The listing builds one solid part. Answer for the finished solid, in the listing's coordinates (mm). A direction names the side the tool comes from. Round coordinates to 2 decimals unless told otherwise and drop trailing zeros. Write each loop counter-clockwise with the first axis right and the second up, starting at its lowest first coordinate (ties: lowest second). Pieces come first, ordered by that corner, then holes. Notation, with made-up numbers: (-1.75, 72.25) - (21.25, 72.25) arc R6 cw to (21.25, 77.25) - close; hole circle Ø9 at (-17.5, 67). An arc over 180 degrees is marked (long way). Answer in a Markdown table with one row per item.
from build123d import *
from OCP.BRepFilletAPI import BRepFilletAPI_MakeChamfer

# Parameters (mm, degrees)
EXTRUDE_1_DEPTH         = 8
CHAMFER_12_SIZE         = 7
CHAMFER_12_SIZE2        = 5
HOLE_WIZARD_M2_22_D     = 2.3
HOLE_WIZARD_M2_22_DEPTH = 3.5
HOLE_WIZARD_M2_22_TIP   = 0.690989712
SKETCH_11_R             = 30
CUT_EXTRUDE_1_DEPTH     = 1.5
EXTRUDE_5_DEPTH         = 8
EXTRUDE_5_2_DEPTH       = 8
EXTRUDE_5_3_DEPTH       = 8
EXTRUDE_5_4_DEPTH       = 8
CHAMFER_13_SIZE         = 5
CHAMFER_13_SIZE2        = 7
CHAMFER_14_SIZE         = 5
CHAMFER_14_SIZE2        = 7
CHAMFER_15_SIZE         = 7
CHAMFER_15_SIZE2        = 5
CHAMFER_16_SIZE         = 5
CHAMFER_16_SIZE2        = 7
SKETCH_23_W             = 32
SKETCH_23_H             = 72
CUT_EXTRUDE_7_DEPTH     = 1.5
SKETCH_13_W             = 16
SKETCH_13_H             = 24
CUT_EXTRUDE_2_DEPTH     = 1.5


with BuildPart() as part:
    # Эскиз1 → Бобышка-Вытянуть1 (new body)
    with BuildSketch(Plane.XY):
        with BuildLine():
            Line((28.8, 21.6), (0, 60))
            Line((0, 60), (-28.8, 21.6))
            ThreePointArc((-28.8, 21.6), (-36, 0), (-28.8, -21.6))
            Line((-28.8, -21.6), (0, -60))
            Line((0, -60), (28.8, -21.6))
            ThreePointArc((28.8, -21.6), (36, 0), (28.8, 21.6))
        make_face()
        with BuildLine():
            ThreePointArc((4.1408267, 28.197580645), (0, -28.5), (-4.1408267, 28.197580645))
            ThreePointArc((-4.1408267, 28.197580645), (0, 26), (4.1408267, 28.197580645))
        make_face(mode=Mode.SUBTRACT)
    extrude(amount=EXTRUDE_1_DEPTH)

    # Фаска12: one chamfer whose edges measure the first distance from different faces: ONE call of the kernel's chamfer builder (chamfer() names one face for all edges)
    chamfer_12_edges_1 = [part.edges().sort_by_distance(p)[0] for p in [
        (14.4, 40.8, 0),
    ]]
    chamfer_12_side_1 = [part.faces().sort_by_distance(p)[0] for p in [
        (14.4, 40.8, 4),
    ]]
    chamfer_12_edges_2 = [part.edges().sort_by_distance(p)[0] for p in [
        (36, 0, 0),
    ]]
    chamfer_12_side_2 = [part.faces().sort_by_distance(p)[0] for p in [
        (36, 0, 4),
    ]]
    chamfer_12_edges_3 = [part.edges().sort_by_distance(p)[0] for p in [
        (14.4, -40.8, 0),
    ]]
    chamfer_12_side_3 = [part.faces().sort_by_distance(p)[0] for p in [
        (14.4, -40.8, 4),
    ]]
    chamfer_12_edges_4 = [part.edges().sort_by_distance(p)[0] for p in [
        (-14.4, -40.8, 0),
    ]]
    chamfer_12_side_4 = [part.faces().sort_by_distance(p)[0] for p in [
        (-14.4, -40.8, 4),
    ]]
    chamfer_12_edges_5 = [part.edges().sort_by_distance(p)[0] for p in [
        (-36, 0, 0),
    ]]
    chamfer_12_side_5 = [part.faces().sort_by_distance(p)[0] for p in [
        (-36, 0, 4),
    ]]
    chamfer_12_edges_6 = [part.edges().sort_by_distance(p)[0] for p in [
        (-14.4, 40.8, 0),
    ]]
    chamfer_12_side_6 = [part.faces().sort_by_distance(p)[0] for p in [
        (-14.4, 40.8, 4),
    ]]
    chamfer_12 = BRepFilletAPI_MakeChamfer(part.part.solid().wrapped)
    for e in chamfer_12_edges_1:
        chamfer_12.Add(CHAMFER_12_SIZE, CHAMFER_12_SIZE2, e.wrapped, chamfer_12_side_1[0].wrapped)  # the first distance lies on this face
    for e in chamfer_12_edges_2:
        chamfer_12.Add(CHAMFER_12_SIZE, CHAMFER_12_SIZE2, e.wrapped, chamfer_12_side_2[0].wrapped)  # the first distance lies on this face
    for e in chamfer_12_edges_3:
        chamfer_12.Add(CHAMFER_12_SIZE, CHAMFER_12_SIZE2, e.wrapped, chamfer_12_side_3[0].wrapped)  # the first distance lies on this face
    for e in chamfer_12_edges_4:
        chamfer_12.Add(CHAMFER_12_SIZE, CHAMFER_12_SIZE2, e.wrapped, chamfer_12_side_4[0].wrapped)  # the first distance lies on this face
    for e in chamfer_12_edges_5:
        chamfer_12.Add(CHAMFER_12_SIZE, CHAMFER_12_SIZE2, e.wrapped, chamfer_12_side_5[0].wrapped)  # the first distance lies on this face
    for e in chamfer_12_edges_6:
        chamfer_12.Add(CHAMFER_12_SIZE, CHAMFER_12_SIZE2, e.wrapped, chamfer_12_side_6[0].wrapped)  # the first distance lies on this face
    add(Compound.cast(chamfer_12.Shape()), mode=Mode.REPLACE)

    # Hole Wizard M2.22
    with Locations(Plane.XY.offset(8)):
        with Locations((0, 31), (-11, -31), (11, -31)):
            Hole(HOLE_WIZARD_M2_22_D / 2, depth=HOLE_WIZARD_M2_22_DEPTH)
            with Locations((0, 0, -(HOLE_WIZARD_M2_22_DEPTH + HOLE_WIZARD_M2_22_TIP / 2))):  # 118° drill point
                Cone(0, HOLE_WIZARD_M2_22_D / 2, HOLE_WIZARD_M2_22_TIP, mode=Mode.SUBTRACT)

    # Эскиз11 → Вырез-Вытянуть1 (cut)
    with BuildSketch(Plane(origin=(0, 0, 0), x_dir=(-1, 0, 0), z_dir=(0, 0, -1))):
        Circle(SKETCH_11_R)
    extrude(amount=-CUT_EXTRUDE_1_DEPTH, mode=Mode.SUBTRACT)


with BuildPart() as body_2:
    # Эскиз17 → Бобышка-Вытянуть5 (new body)
    with BuildSketch(Plane(origin=(0, 0, 8), x_dir=(-1, 0, 0), z_dir=(0, 0, -1))):
        with BuildLine():
            Line((25.238858928, -18), (28.902564257, -20.612903226))
            Line((28.902564257, -20.612903226), (53.902564257, 8.387096774))
            Line((53.902564257, 8.387096774), (30.528334189, 5.387096774))
            ThreePointArc((30.528334189, 5.387096774), (30.236303195, -6.838564841), (25.238858928, -18))
        make_face()
    extrude(amount=EXTRUDE_5_DEPTH)

    # Фаска13
    chamfer_13_edges = [body_2.edges().sort_by_distance(p)[0] for p in [
        (-41.402564257, -6.112903226, 0),
    ]]
    chamfer_13_side = [body_2.faces().sort_by_distance(p)[0] for p in [
        (-37.369612162, -3.153009871, 0),
    ]]
    chamfer(chamfer_13_edges, length=CHAMFER_13_SIZE, length2=CHAMFER_13_SIZE2, reference=chamfer_13_side[0])


with BuildPart() as body_3:
    # Эскиз17 → Extrude 5 2 (new body)
    with BuildSketch(Plane(origin=(0, 0, 8), x_dir=(-1, 0, 0), z_dir=(0, 0, -1))):
        with BuildLine():
            Line((-28.902564257, -20.612903226), (-25.238858928, -18))
            ThreePointArc((-25.238858928, -18), (-30.236303195, -6.838564841), (-30.528334189, 5.387096774))
            Line((-30.528334189, 5.387096774), (-53.902564257, 8.387096774))
            Line((-53.902564257, 8.387096774), (-28.902564257, -20.612903226))
        make_face()
    extrude(amount=EXTRUDE_5_2_DEPTH)

    # Фаска14
    chamfer_14_edges = [body_3.edges().sort_by_distance(p)[0] for p in [
        (41.402564257, -6.112903226, 0),
    ]]
    chamfer_14_side = [body_3.faces().sort_by_distance(p)[0] for p in [
        (37.369612162, -3.153009871, 0),
    ]]
    chamfer(chamfer_14_edges, length=CHAMFER_14_SIZE, length2=CHAMFER_14_SIZE2, reference=chamfer_14_side[0])


with BuildPart() as body_4:
    # Эскиз17 → Extrude 5 3 (new body)
    with BuildSketch(Plane(origin=(0, 0, 8), x_dir=(-1, 0, 0), z_dir=(0, 0, -1))):
        with BuildLine():
            ThreePointArc((23.416468646, 20.314255983), (27.763165047, 13.791543298), (30.334880827, 6.387096774))
            Line((30.334880827, 6.387096774), (34.73833127, 7.314255983))
            Line((34.73833127, 7.314255983), (42.73833127, 24.314255983))
            Line((42.73833127, 24.314255983), (23.416468646, 20.314255983))
        make_face()
    extrude(amount=EXTRUDE_5_3_DEPTH)

    # Фаска16
    chamfer_16_edges = [body_4.edges().sort_by_distance(p)[0] for p in [
        (-38.73833127, 15.814255983, 0),
    ]]
    chamfer_16_side = [body_4.faces().sort_by_distance(p)[0] for p in [
        (-33.199864657, 16.363314329, 0),
    ]]
    chamfer(chamfer_16_edges, length=CHAMFER_16_SIZE, length2=CHAMFER_16_SIZE2, reference=chamfer_16_side[0])


with BuildPart() as body_5:
    # Эскиз17 → Extrude 5 4 (new body)
    with BuildSketch(Plane(origin=(0, 0, 8), x_dir=(-1, 0, 0), z_dir=(0, 0, -1))):
        with BuildLine():
            Line((-34.73833127, 7.314255983), (-30.334880827, 6.387096774))
            ThreePointArc((-30.334880827, 6.387096774), (-27.763165047, 13.791543298), (-23.416468646, 20.314255983))
            Line((-23.416468646, 20.314255983), (-42.73833127, 24.314255983))
            Line((-42.73833127, 24.314255983), (-34.73833127, 7.314255983))
        make_face()
    extrude(amount=EXTRUDE_5_4_DEPTH)

    # Фаска15
    chamfer_15_edges = [body_5.edges().sort_by_distance(p)[0] for p in [
        (38.73833127, 15.814255983, 0),
    ]]
    chamfer_15_side = [body_5.faces().sort_by_distance(p)[0] for p in [
        (38.73833127, 15.814255983, 4),
    ]]
    chamfer(chamfer_15_edges, length=CHAMFER_15_SIZE, length2=CHAMFER_15_SIZE2, reference=chamfer_15_side[0])


with BuildPart() as body_2_1:
    add(body_2.part)

    # Combine 2: union body 3, body 5, body 4, part
    add(body_3.part)
    add(body_5.part)
    add(body_4.part)
    add(part.part)

    # Эскиз23 → Вырез-Вытянуть7 (cut)
    with BuildSketch(Plane.XY.offset(8)):
        Rectangle(SKETCH_23_W, SKETCH_23_H)
    extrude(amount=-CUT_EXTRUDE_7_DEPTH, mode=Mode.SUBTRACT)

    # Эскиз13 → Вырез-Вытянуть2 (cut)
    with BuildSketch(Plane.XY.offset(8)):
        with Locations((0, -48)):
            Rectangle(SKETCH_13_W, SKETCH_13_H)
    extrude(amount=-CUT_EXTRUDE_2_DEPTH, mode=Mode.SUBTRACT)


solid = body_2_1.part
(1) Section A-A (x = -17.5) is taken. Give the vertices of the cut face in (y, z).
Checked values:
| item | result |
|---|---|
| outline | (-36.67, 7) - (-28.33, 0) - (-24.37, 0) - (-24.37, 1.5) - (-22.49, 1.5) - (-22.49, 8) - (-36.67, 8) - close; (22.49, 1.5) - (24.37, 1.5) - (24.37, 0) - (28.33, 0) - (36.67, 7) - (36.67, 8) - (22.49, 8) - close |
(2) For a pull along X with two mould halves and no side action, classify faces 4 (the flat face through (0, 27, 1.5)), 5 (the cylindrical face through (-30.084, -19.773, 7.493)), 6 (the flat face through (0, 33, 6.5)), 7 (the conical face through (28.07, -18.22, 3.45)) as pulls with the +X half, pulls with the -X half, needs draft (parallel to the pull), parting line crosses it, or undercut.
Checked values:
| item | result |
|---|---|
| face 4 | undercut |
| face 5 | pulls with the -X half |
| face 6 | undercut |
| face 7 | pulls with the +X half |
(3) Find the intervals of material crossed by line 1 (Y direction, x = 11, z = 5.4); line 2 (Y direction, x = 1, z = 5.25); line 3 (X direction, y = -35.5, z = 7) (3 decimals), in increasing order.
Checked values:
| item | result |
|---|---|
| line 1 | y = -43.43 to -32.15, -29.85 to -26.29, 26.29 to 43.43 |
| line 2 | y = -56.58 to -28.48, 26.1 to 30.43, 31.57 to 56.58 |
| line 3 | x = -18.375 to -16, 16 to 18.375 |
(4) For faces 1 (the flat face through (33, 22.3, 4.1)), 2 (the cylindrical face through (29.97, 1.32, 0.74)), 3 (the cylindrical face through (1.195, -28.475, 4.704)), determine the directions among +Z, -Z, +X, -X, +Y, -Y from which every point of the face is accessible in a straight line to the end or side of a thin tool.
Checked values:
| item | result |
|---|---|
| face 1 | -Z, +Y |
| face 2 | -Z |
| face 3 | +Z, -Z |
(5) Section B-B (y = 0) is taken. Give the vertices of the cut face in (x, z), and give its area (3 significant figures).
Checked values:
| item | result |
|---|---|
| outline | (-46.67, 7) - (-40.07, 0) - (-30, 0) - (-30, 1.5) - (-28.5, 1.5) - (-28.5, 8) - (-46.67, 8) - close; (28.5, 1.5) - (30, 1.5) - (30, 0) - (40.07, 0) - (46.67, 7) - (46.67, 8) - (28.5, 8) - close |
| area | 240 mm2 |
(6) Flat-ended cylindrical pins translate along their axes: pin 1 (2 mm diameter, centred on y = -39.5, z = 3, fed in from -X); pin 2 (1.2 mm diameter, centred on y = 29, z = 7, fed in from +X); pin 3 (3.5 mm diameter, centred on x = 3.5, y = 28.5, fed in from +Z). Find the tip coordinate at first contact, or state that the pin passes through.
Checked values:
| item | result |
|---|---|
| pin 1 | stops at x = -12.97 |
| pin 2 | stops at x = 23.7 |
| pin 3 | stops at z = 6.5 |
